```python
from build123d import *

# Parameters (mm, degrees)
ESQUISSE2_R                  = 2.5
ENL_V_MAT_EXTRU_1_DEPTH      = 14
ENL_V_MAT_EXTRU_1_DEPTH_BACK = 14


with BuildPart() as part:
    # Esquisse1 → Révolution1 (revolve)
    with BuildSketch(Plane.XY):
        Polygon((0, 0), (0, -100), (-3, -100), (-3, -90), (-13, -90), (-13, -70), (-3, -70), (-3, 0), align=None)
    revolve(axis=Axis((0, 0, 0), (0, -1, 0)))

    # Esquisse2 → Enlèv. mat.-Extru.1 (cut, two sides)
    with BuildSketch(Plane.XY) as enl_v_mat_extru_1_sk:
        with Locations((0, -5)):
            Circle(ESQUISSE2_R)
    extrude(amount=ENL_V_MAT_EXTRU_1_DEPTH, mode=Mode.SUBTRACT)
    extrude(enl_v_mat_extru_1_sk.sketch, amount=-ENL_V_MAT_EXTRU_1_DEPTH_BACK, mode=Mode.SUBTRACT)


solid = part.part
```
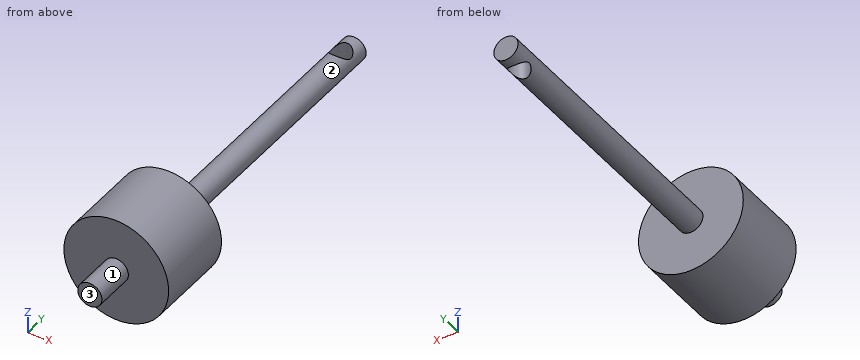
Geometry check sheet. Reference: the model listing, model coordinates, mm. Face numbers are marked on the shaded views. A direction names the side the tool comes from. Give positions to 0.01 mm unless a question says otherwise; leave off trailing zeros. Order: outer loops, then holes, each group sorted by start corner. A loop starts at its lowest first (then second) coordinate and runs counter-clockwise, first axis right, second up. Notation, with made-up numbers: (21.5, 66.25) - (41.5, 66.25) arc R10 ccw to (41.5, 73.25) - close; hole circle Ø9 at (89.5, -32.75). An arc over 180 degrees is marked (long way). Answer in a Markdown table with one row per item. Add a question column.
Q1. Material ranges on probe 1 along Y at (x, z) = (0, 1.75); probe 2 along X at (y, z) = (-5, 0.25); probe 3 along Y at (x, z) = (-10, 4), recorded low to high. Write a range as from..to.
Q2. Gauge pin test, flat ends, axial feed: pin 1 (1 mm diameter, centred on y = -56, z = 0, fed in from -X); pin 2 (12 mm diameter, centred on x = -9.5, y = -70.5, fed in from -Z); pin 3 (8 mm diameter, centred on y = -83, z = 7.5, fed in from -X); pin 4 (10 mm diameter, centred on y = -43, z = 8.5, fed in from -X). Record the tip position at first contact, or that the pin passes through.
Q3. Cross-section at A-A, the plane x = 0. Enter the section's corners in (y, z).
Q4. Tool access check on the marked faces 1, 2 and 3. Record the directions out of +Z, -Z, +X, -X, +Y, -Y that give a thin tool (end or side, any length) a straight path to the whole face; none if there is none.
Q5. Cross-section at B-B, the plane z = 0. Enter the section's corners in (x, y).
Q6. Cross-section at D-D, the plane y = -5. Enter the section's corners in (x, z), then the cut area to 3 significant figures.
Q7. Cross-section at C-C, the plane y = -60. Enter the section's corners in (x, z).
Check values:
| question | item | result |
|---|---|---|
| 1 | probe 1 | y = -100..-7.5, -2.5..0 |
| 1 | probe 2 | x = -2.99..-2.5, 2.5..2.99 |
| 1 | probe 3 | y = -90..-70 |
| 2 | pin 1 | stops at x = -3 |
| 2 | pin 2 | stops at z = -12.52 |
| 2 | pin 3 | stops at x = -12.52 |
| 2 | pin 4 | passes through |
| 3 | outline | (-100, -3) - (-90, -3) - (-90, -13) - (-70, -13) - (-70, -3) - (-7.5, -3) - (-7.5, 3) - (-70, 3) - (-70, 13) - (-90, 13) - (-90, 3) - (-100, 3) - close; (-2.5, -3) - (0, -3) - (0, 3) - (-2.5, 3) - close |
| 4 | face 1 | -Y |
| 4 | face 2 | +Y |
| 4 | face 3 | +Z, -Z, +X, -X, -Y |
| 5 | outline | (-13, -90) - (-3, -90) - (-3, -100) - (3, -100) - (3, -90) - (13, -90) - (13, -70) - (3, -70) - (3, 0) - (-3, 0) - (-3, -70) - (-13, -70) - close; hole circle Ø5 at (0, -5) |
| 6 | outline | (-2.5, -1.66) - (-2.5, 1.66) arc R3 ccw to start; (2.5, -1.66) arc R3 ccw to (2.5, 1.66) - close |
| 6 | area | 2.25 mm^2 |
| 7 | outline | circle Ø6 at (0, 0) |
